```python
from build123d import *

# Parameters (mm, degrees)
SKETCH1_R           = 100
BOSS_EXTRUDE1_DEPTH = 3
SKETCH2_R           = 5
BOSS_EXTRUDE2_DEPTH = 50
SKETCH3_R           = 10
BOSS_EXTRUDE3_DEPTH = 10


with BuildPart() as part:
    # Sketch1 → Boss-Extrude1 (new body)
    with BuildSketch(Plane(origin=(0, 0, 0), x_dir=(1, 0, 0), z_dir=(0, 1, 0))):
        with Locations(Location((0, 0, 0), (0, 0, 270))):
            Circle(SKETCH1_R)
    boss_extrude1 = extrude(amount=BOSS_EXTRUDE1_DEPTH)

    # Sketch2 → Boss-Extrude2 (add)
    with BuildSketch(Plane(origin=(0, 3, 0), x_dir=(1, 0, 0), z_dir=(0, 1, 0))):
        with Locations(Location((-90, 0, 0), (0, 0, 270))):
            Circle(SKETCH2_R)
        with Locations(Location((0, 90, 0), (0, 0, 270))):
            Circle(SKETCH2_R)
        with Locations(Location((90, 0, 0), (0, 0, 270))):
            Circle(SKETCH2_R)
        with Locations(Location((0, -90, 0), (0, 0, 270))):
            Circle(SKETCH2_R)
    extrude(amount=BOSS_EXTRUDE2_DEPTH)

    # Mirror1: Boss-Extrude1 across plane
    add(boss_extrude1.mirror(Plane.ZX.offset(28)))

    # Sketch3 → Boss-Extrude3 (add)
    with BuildSketch(Plane(origin=(0, 56, 0), x_dir=(1, 0, 0), z_dir=(0, 1, 0))):
        with Locations(Location((0, 0, 0), (0, 0, 90))):
            Circle(SKETCH3_R)
    extrude(amount=BOSS_EXTRUDE3_DEPTH)


solid = part.part
```
Model file for the job. Use its own axes, mm. A direction names the side the tool comes from. Round coordinates to 2 decimals unless told otherwise and drop trailing zeros. Write each loop counter-clockwise with the first axis right and the second up, starting at its lowest first coordinate (ties: lowest second). Pieces come first, ordered by that corner, then holes. Notation, with made-up numbers: (20, 87.25) -> (61, 87.25) arc R23 cw to (61, 114.25) -> close; hole circle Ø4 at (56.25, 9). An arc over 180 degrees is marked (long way). Answer as CSV lines item,"result".
1. Slice it at A-A, the plane z = 0. List the corners of the cut face in (x, y).
Resolved:
outline,"(-100, 0) -> (100, 0) -> (100, 3) -> (95, 3) -> (95, 53) -> (100, 53) -> (100, 56) -> (10, 56) -> (10, 66) -> (-10, 66) -> (-10, 56) -> (-100, 56) -> (-100, 53) -> (-95, 53) -> (-95, 3) -> (-100, 3) -> close; hole (-85, 3) -> (85, 3) -> (85, 53) -> (-85, 53) -> close"
2. Mould opens along Y. For faces 5 (the face through (-1.915, 27.65, 94.619)), 6 (the face through (1, 53, -1)), 7 (the face through (1, 0, -1)), 8 (the face through (30.04, 1.48, 95.38)) say: +Y half, -Y half, draft (parallel to the pull), parting line (faces both ways), or undercut.
Resolved:
face 5,"undercut"
face 6,"undercut"
face 7,"-Y half"
face 8,"draft"
3. Pin check, flat tips, straight feed: pin 1 Ø10 at (x, y) = (-68, 53) entering from -Z; pin 2 Ø1.5 at (x, z) = (3.5, -42.5) entering from +Y; pin 3 Ø12 at (y, z) = (9.5, -20) entering from +X; pin 4 Ø12 at (x, y) = (-6.5, 44) entering from +Z. Stop position of each tip, or through.
Resolved:
pin 1,"z = -77.66"
pin 2,"y = 56"
pin 3,"through"
pin 4,"z = 94.97"
4. Slice it at B-B, the plane x = 81. List the corners of the cut face in (y, z), plus the area to 3 significant figures.
Resolved:
outline,"(0, -58.64) -> (3, -58.64) -> (3, 58.64) -> (0, 58.64) -> close; (53, -58.64) -> (56, -58.64) -> (56, 58.64) -> (53, 58.64) -> close"
area,"704 mm²"
5. Tool access for faces 1 (the face through (9.76, 60.93, 2.17)), 2 (the face through (30.04, 54.52, 95.38)), 3 (the face through (0, 66, 0)), 4 (the face through (85.12, 27.65, -1.08)): list every direction of +Z, -Z, +X, -X, +Y, -Y with a clear straight run to the whole face (end or side of a thin tool).
Resolved:
face 1,"+Y"
face 2,"+Y, -Y"
face 3,"+Z, -Z, +X, -X, +Y"
face 4,"none"
6. Slice it at C-C, the plane x = 0. List the corners of the cut face in (y, z).
Resolved:
outline,"(0, -100) -> (3, -100) -> (3, -95) -> (53, -95) -> (53, -100) -> (56, -100) -> (56, -10) -> (66, -10) -> (66, 10) -> (56, 10) -> (56, 100) -> (53, 100) -> (53, 95) -> (3, 95) -> (3, 100) -> (0, 100) -> close; hole (3, -85) -> (53, -85) -> (53, 85) -> (3, 85) -> close"
7. Drill centre lines: line 1 (Y direction, x = 82.5, z = 24); line 2 (Z direction, x = 3.5, y = 47.5); line 3 (Z direction, x = -4, y = 11.5). Where is each one in solid material? Low to high.
Resolved:
line 1,"0 to 3, 53 to 56"
line 2,"-93.57 to -86.43, 86.43 to 93.57"
line 3,"-93 to -87, 87 to 93"
8. Slice it at D-D, the plane z = 80.5. List the corners of the cut face in (x, y), plus the area to 3 significant figures.
Resolved:
outline,"(-59.33, 0) -> (59.33, 0) -> (59.33, 3) -> (-59.33, 3) -> close; (-59.33, 53) -> (59.33, 53) -> (59.33, 56) -> (-59.33, 56) -> close"
area,"712 mm²"
